Source: CAD feature listing. Evaluate the final solid. Frame: model axes, mm. Give positions to 0.01 mm unless a question says otherwise; leave off trailing zeros. Write each loop counter-clockwise with the first axis right and the second up, starting at its lowest first coordinate (ties: lowest second). Pieces come first, ordered by that corner, then holes. Notation, with made-up numbers: M 16.5,49.25 L 45.5,49.25 A7 cw 45.5,55.25 Z; hole C 38,58 d4. An arc over 180 degrees is marked long. Return JSON: item names as keys, results as strings.
```python
from build123d import *

# Parameters (mm, degrees)
F0_R     = 13.97
F1_DEPTH = 44.45
F4_DEPTH = 11.6078


with BuildPart() as f1:
    # F0 (on Front) → F1 (new body)
    with BuildSketch(Plane.XZ):
        Circle(F0_R)
    extrude(amount=F1_DEPTH)

    # F2: F1 across plane


with BuildPart() as f1_1:
    add(f1.part)
    add(f1.part.mirror(Plane.XZ))

    # F3 (on face) → F4 (cut)
    with BuildSketch(Plane(origin=(0, 44.45, 0), x_dir=(-1, 0, 0), z_dir=(0, 1, 0))):
        Polygon((2.044567, 3.151697), (0, 3.175), (-2.0447, 3.175), (-3.556, 0), (-2.008188, -3.175), (0.036512, -3.175), (2.081212, -3.175), (3.556, 0), align=None)
    extrude(amount=-F4_DEPTH, mode=Mode.SUBTRACT)


solid = f1_1.part
```
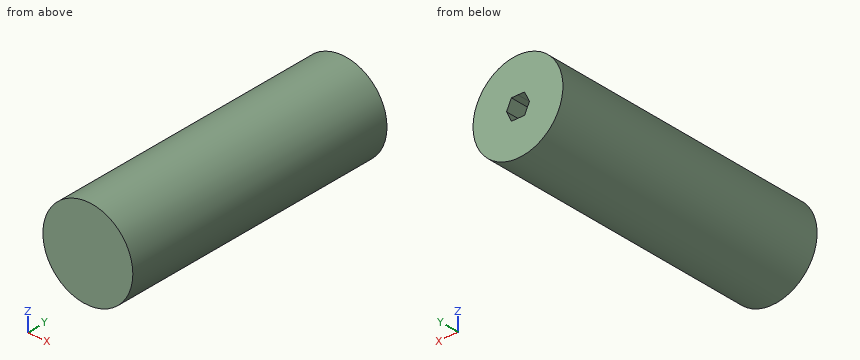
1) Contact query for flat-ended pins moving along their axis: pin 1 Ø4 at (x, y) = (-6.5, -14.5) entering from +Z; pin 2 Ø2 at (y, z) = (16.5, -8.5) entering from +X; pin 3 Ø1 at (x, y) = (1.5, 38.5) entering from -Z; pin 4 Ø1.2 at (x, y) = (0.5, 38) entering from +Z. Output: stop coordinate, or through.
Numbers:
{"pin 1": "stops at z = 13.23", "pin 2": "stops at x = 11.79", "pin 3": "stops at z = -13.93", "pin 4": "stops at z = 13.97"}
2) Cut plane C-C, the plane z = 11.5. Return the cut outline in (x, y), then the cut area to 3 significant figures.
Numbers:
{"outline": "M -7.93,-44.45 L 7.93,-44.45 L 7.93,44.45 L -7.93,44.45 Z", "area": "1,410 mm²"}
3) Line query: line 1 (Y direction, x = -1.5, z = 2.5); line 2 (X direction, y = -25, z = -1); line 3 (Z direction, x = -2.25, y = 5). Output: solid intervals per line, ascending. Write a range as [from, to].
Numbers:
{"line 1": "y = [-44.45, 32.84]", "line 2": "x = [-13.93, 13.93]", "line 3": "z = [-13.79, 13.79]"}
4) Cut plane B-B, the plane x = -7.75. Return the cut outline in (y, z), then the cut area to 3 significant figures.
Numbers:
{"outline": "M -44.45,-11.62 L 44.45,-11.62 L 44.45,11.62 L -44.45,11.62 Z", "area": "2,070 mm²"}
5) Cut plane A-A, the plane y = -36. Return the cut outline in (x, z).
Numbers:
{"outline": "C 0,0 d27.94"}
